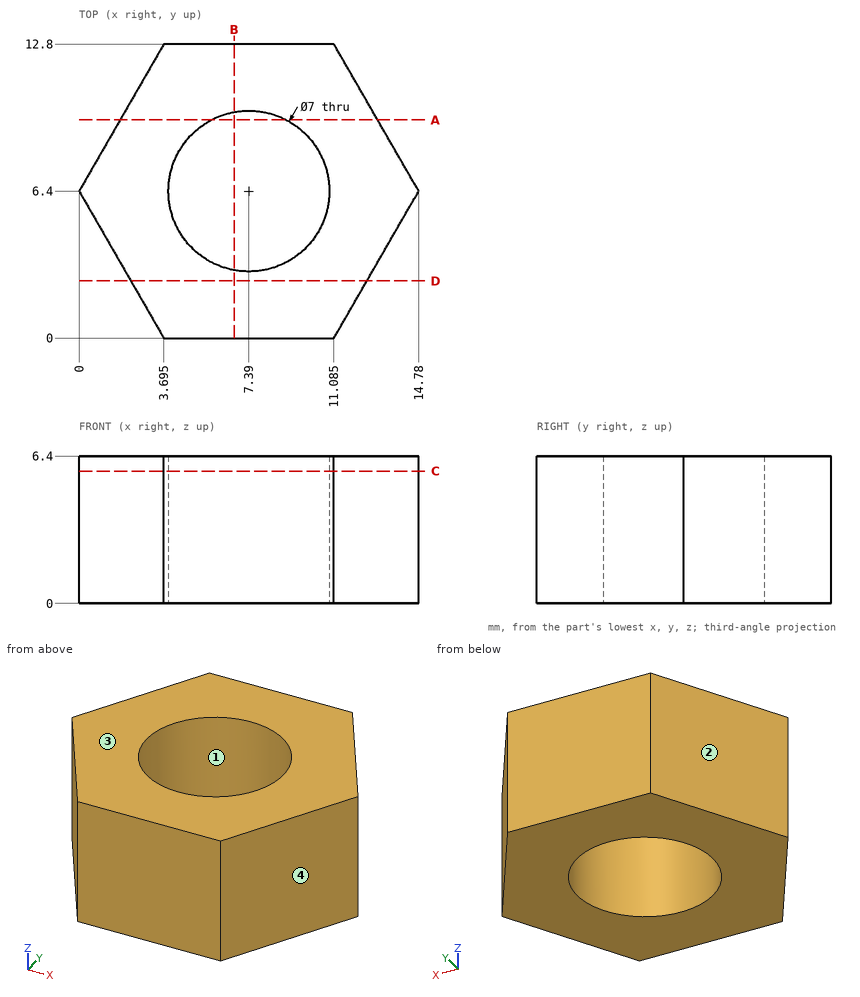
Study the drawing (mm; zero at the part's minimum x, y, z) and answer. Coordinates: 2 decimals unless noted, no trailing zeros. Order: outer loops, then holes, each group sorted by start corner. A loop starts at its lowest first (then second) coordinate and runs counter-clockwise, first axis right, second up. Notation, with made-up numbers: M 40,68 L 70,68 A13 cw 70,72 Z; hole C 67.5,-30 d11. An arc over 180 degrees is marked long. Answer as a JSON object with one key per item and string values. Group by question number.
1. Section B-B on x = 6.75 is taken. Write down the section's boundary in (y, z).
2. Section A-A on y = 9.5 is taken. Write down the section's boundary in (x, z) (1 decimal), then the cut area to 3 significant figures.
3. Determine the mould class of the marked faces 1, 2, 3 and 4 for opening direction X: released by +X, released by -X, zero draft, split by the parting line, or undercut.
4. Section D-D on y = 2.5 is taken. Write down the section's boundary in (x, z), then the cut area to 3 significant figures.
5. Straight lines are drawn through the part: line 1 (X direction, y = 7.75, z = 5); line 2 (X direction, y = 6.75, z = 4); line 3 (Y direction, x = 9.75, z = 2.5) (1 decimal). For each, find the intervals that lie inside material, in ascending order.
6. Section C-C on z = 5.75 is taken. Write down the section's boundary in (x, y) (1 decimal), then the cut area to 3 significant figures.
7. Flat-ended cylindrical pins translate along their axes: P1, Ø5.5, axis at x = 7.39, y = 6.4, coming from the +Z side; P2, Ø1.5, axis at x = 1.5, z = 4.5, coming from the -Y side. Find the tip coordinate at first contact, or state that the pin passes through.
Values follow:
{
 "1": {"outline": "M 0,0 L 2.96,0 L 2.96,6.4 L 0,6.4 Z; M 9.84,0 L 12.8,0 L 12.8,6.4 L 9.84,6.4 Z"},
 "2": {"outline": "M 1.8,0 L 5.8,0 L 5.8,6.4 L 1.8,6.4 Z; M 9,0 L 13,0 L 13,6.4 L 9,6.4 Z", "area": "50.9 mm2"},
 "3": {"face 1": "undercut", "face 2": "released by -X", "face 3": "zero draft", "face 4": "released by +X"},
 "4": {"outline": "M 2.25,0 L 12.53,0 L 12.53,6.4 L 2.25,6.4 Z", "area": "65.8 mm2"},
 "5": {"line 1": "0.78 to 4.16, 10.62 to 14", "line 2": "0.2 to 3.91, 10.87 to 14.58", "line 3": "0 to 3.8, 9 to 12.8"},
 "6": {"outline": "M 0,6.4 L 3.7,0 L 11.1,0 L 14.8,6.4 L 11.1,12.8 L 3.7,12.8 Z; hole C 7.4,6.4 d7", "area": "103 mm2"},
 "7": {"P1": "through", "P2": "y = 2.5"}
}
